from build123d import *

# Parameters (mm, degrees)
EXTRUDE_1_DEPTH              = 20
HOLE_WIZARD_M6_1_D           = 6.6
HOLE_WIZARD_M6_1_CBORE_D     = 12
HOLE_WIZARD_M6_1_CBORE_DEPTH = 0.5
HOLE_WIZARD_M6_2_D           = 6.6
HOLE_WIZARD_M6_2_CBORE_D     = 12
HOLE_WIZARD_M6_2_CBORE_DEPTH = 0.5
FILLET_1_R                   = 2


with BuildPart() as part:
    # 草图1 → 凸台-拉伸1 (new, symmetric)
    with BuildSketch(Plane.XY):
        Polygon((0, 21), (0, 0), (21, 0), (21, 4.5), (4.5, 4.5), (4.5, 21), align=None)
    extrude(amount=EXTRUDE_1_DEPTH, both=True)

    # M6 六角头螺栓的柱形沉头孔1 (through all)
    with Locations(Plane(origin=(0, 4.5, 0), x_dir=(1, 0, 0), z_dir=(0, 1, 0))):
        with Locations((12.75, 12), (12.75, -12)):
            CounterBoreHole(HOLE_WIZARD_M6_1_D / 2, HOLE_WIZARD_M6_1_CBORE_D / 2, HOLE_WIZARD_M6_1_CBORE_DEPTH)

    # M6 六角头螺栓的柱形沉头孔2 (through all)
    with Locations(Plane(origin=(4.5, 0, 0), x_dir=(0, 0, -1), z_dir=(1, 0, 0))):
        with Locations((12, 12.75), (-12, 12.75)):
            CounterBoreHole(HOLE_WIZARD_M6_2_D / 2, HOLE_WIZARD_M6_2_CBORE_D / 2, HOLE_WIZARD_M6_2_CBORE_DEPTH)

    # 圆角1
    fillet_1_edges = [part.edges().sort_by_distance(p)[0] for p in [
        (21, 2.25, 20),
        (2.25, 21, 20),
        (21, 2.25, -20),
        (2.25, 21, -20),
    ]]
    fillet(fillet_1_edges, radius=FILLET_1_R)


solid = part.part
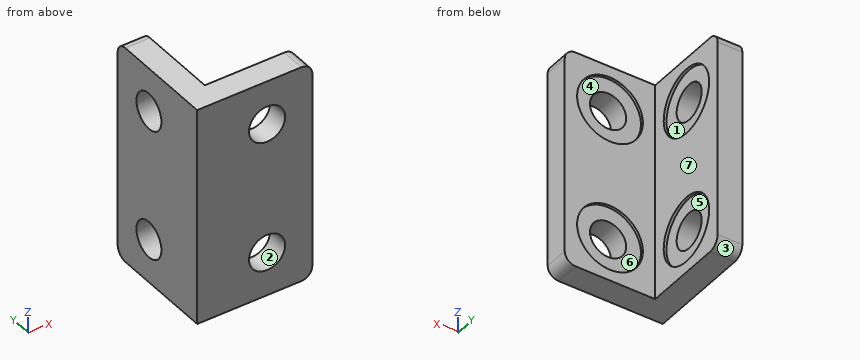
Verification items for the finished model (mm, model axes). Face numbers are marked on the shaded views. A direction names the side the tool comes from. Give positions to 0.01 mm unless a question says otherwise; leave off trailing zeros. Loops run counter-clockwise (first coordinate to the right, second up) from the corner with the lowest first, then second, coordinate; pieces in that order, holes last. Notation, with made-up numbers: (72, 67.5) - (120, 67.5) arc R16 cw to (120, 79.5) - close; hole circle Ø10 at (-6, -27.5). An arc over 180 degrees is marked (long way). Write each question's results on one line, items separated by ' | '.
1) Material ranges on L1, parallel to Z at x = 12.75, y = 4.35; L2, parallel to Z at x = 12.75, y = 2.65; L3, parallel to Y at x = 2.7, z = -12, recorded low to high. Write a range as from..to.
Solution:
L1: -20..-18, -6..6, 18..20 | L2: -20..-15.3, -8.7..8.7, 15.3..20 | L3: 0..9.45, 16.05..21
2) Tool access check on the marked faces 5, 6 and 7. Record the directions out of +Z, -Z, +X, -X, +Y, -Y that give a thin tool (end or side, any length) a straight path to the whole face; none if there is none.
Solution:
face 5: +X | face 6: +Y | face 7: +Z, -Z, +X, +Y
3) Mould release check, pull along X, two halves, no side actions. Record for the marked faces 1, 2, 3 and 4: pulls with the +X half, pulls with the -X half, needs draft (parallel to the pull), parting line crosses it, or undercut.
Solution:
face 1: pulls with the +X half | face 2: undercut | face 3: needs draft | face 4: undercut
4) Sectioned sample at A-A on z = 12. Record the boundary of the cut face in (x, y).
Solution:
outline: (0, 0) - (9.45, 0) - (9.45, 4) - (6.75, 4) - (6.75, 4.5) - (4.5, 4.5) - (4.5, 6.75) - (4, 6.75) - (4, 9.45) - (0, 9.45) - close; (0, 16.05) - (4, 16.05) - (4, 18.75) - (4.5, 18.75) - (4.5, 21) - (0, 21) - close; (16.05, 0) - (21, 0) - (21, 4.5) - (18.75, 4.5) - (18.75, 4) - (16.05, 4) - close
5) Sectioned sample at B-B on x = 12.75. Record the boundary of the cut face in (y, z).
Solution:
outline: (0, -20) - (4.5, -20) - (4.5, -18) - (4, -18) - (4, -15.3) - (0, -15.3) - close; (0, -8.7) - (4, -8.7) - (4, -6) - (4.5, -6) - (4.5, 6) - (4, 6) - (4, 8.7) - (0, 8.7) - close; (0, 15.3) - (4, 15.3) - (4, 18) - (4.5, 18) - (4.5, 20) - (0, 20) - close
6) Sectioned sample at D-D on x = 1.75. Record the boundary of the cut face in (y, z).
Solution:
outline: (0, -20) - (19, -20) arc R2 ccw to (21, -18) - (21, 18) arc R2 ccw to (19, 20) - (0, 20) - close; hole circle Ø6.6 at (12.75, -12); hole circle Ø6.6 at (12.75, 12)
7) Depth check by flat-ended pin: P1, Ø7.5, axis at y = 12.75, z = -12, coming from the +X side; P2, Ø7.5, axis at x = 12.75, z = -12, coming from the +Y side; P3, Ø3.5, axis at x = 13, z = -11, coming from the +Y side; P4, Ø3, axis at x = 8, z = -15, coming from the +Y side. Enter the tip coordinate at first touch or a pass-through.
Solution:
P1: x = 4 | P2: y = 4 | P3: through | P4: y = 4.5
